from build123d import *

# Parameters (mm, degrees)
BOSS_EXTRUDE1_DEPTH     = 7
CUT_EXTRUDE1_DEPTH      = 3
CUT_EXTRUDE2_DEPTH      = 59.755326779
CUT_EXTRUDE2_DEPTH_BACK = 1
SKETCH5_W               = 5.5
SKETCH5_H               = 5.5
BOSS_EXTRUDE2_DEPTH     = 7
CUT_LOFT3_START         = -28.140767726
CUT_LOFT3_DEPTH         = 25.989204331


# Read off the part's stored shape, not the designer's step: Cut-Loft3
with BuildPart() as part:
    # Sketch1 → Boss-Extrude1 (new body)
    with BuildSketch(Plane(origin=(0, 0, 0), x_dir=(1, 0, 0), z_dir=(0, 1, 0))):
        with BuildLine():
            Line((-56.7108806, 8.042770274), (-56.7108806, 6.805307476))
            Line((-56.7108806, 6.805307476), (51.827852841, 6.805307476))
            Line((51.827852841, 6.805307476), (51.827852841, 8.042770274))
            add(Edge.make_bspline(
                [(51.827852841, 8.042770274), (43.440678216, 9.870534091), (30.144344491, 11.93787877), (11.99631981, 12.860332352), (2.722791962, 12.844934175), (-2.44151388, 12.817702683)],
                knots=[0, 0, 0, 0, 0.47203113, 0.735860593, 1, 1, 1, 1], degree=3))
            add(Edge.make_bspline(
                [(-56.7108806, 8.042770274), (-48.323705975, 9.870534091), (-35.02737225, 11.93787877), (-16.87934757, 12.860332352), (-7.605819721, 12.844934175), (-2.44151388, 12.817702683)],
                knots=[0, 0, 0, 0, 0.47203113, 0.735860593, 1, 1, 1, 1], degree=3))
        make_face()
        with BuildLine():
            Line((51.827852841, 6.805307476), (-56.7108806, 6.805307476))
            Line((-56.7108806, 6.805307476), (-56.7108806, -1.957229726))
            add(Edge.make_bspline(
                [(-56.7108806, -1.957229726), (-48.323705975, -0.129465909), (-35.02737225, 1.93787877), (-16.87934757, 2.860332352), (-7.605819721, 2.844934175), (-2.44151388, 2.817702683)],
                knots=[0, 0, 0, 0, 0.47203113, 0.735860593, 1, 1, 1, 1], degree=3))
            add(Edge.make_bspline(
                [(51.827852841, -1.957229726), (43.440678216, -0.129465909), (30.144344491, 1.93787877), (11.99631981, 2.860332352), (2.722791962, 2.844934175), (-2.44151388, 2.817702683)],
                knots=[0, 0, 0, 0, 0.47203113, 0.735860593, 1, 1, 1, 1], degree=3))
            Line((51.827852841, -1.957229726), (51.827852841, 6.805307476))
        make_face()
        with BuildLine():
            add(Edge.make_bspline(
                [(-56.7108806, -1.957229726), (-48.323705975, -0.129465909), (-35.02737225, 1.93787877), (-16.87934757, 2.860332352), (-7.605819721, 2.844934175), (-2.44151388, 2.817702683)],
                knots=[0, 0, 0, 0, 0.47203113, 0.735860593, 1, 1, 1, 1], degree=3))
            Line((-56.7108806, -1.957229726), (-56.7108806, -3.957229726))
            add(Edge.make_bspline(
                [(-56.7108806, -3.957229726), (-48.323705975, -2.129465909), (-35.02737225, -0.06212123), (-16.87934757, 0.860332352), (-7.605819721, 0.844934175), (-2.44151388, 0.817702683)],
                knots=[0, 0, 0, 0, 0.47203113, 0.735860593, 1, 1, 1, 1], degree=3))
            add(Edge.make_bspline(
                [(51.827852841, -3.957229726), (43.440678216, -2.129465909), (30.144344491, -0.06212123), (11.99631981, 0.860332352), (2.722791962, 0.844934175), (-2.44151388, 0.817702683)],
                knots=[0, 0, 0, 0, 0.47203113, 0.735860593, 1, 1, 1, 1], degree=3))
            Line((51.827852841, -3.957229726), (51.827852841, -1.957229726))
            add(Edge.make_bspline(
                [(51.827852841, -1.957229726), (43.440678216, -0.129465909), (30.144344491, 1.93787877), (11.99631981, 2.860332352), (2.722791962, 2.844934175), (-2.44151388, 2.817702683)],
                knots=[0, 0, 0, 0, 0.47203113, 0.735860593, 1, 1, 1, 1], degree=3))
        make_face()
        with BuildLine():
            Line((-56.7108806, 10.042770274), (-56.7108806, 8.042770274))
            add(Edge.make_bspline(
                [(-56.7108806, 8.042770274), (-48.323705975, 9.870534091), (-35.02737225, 11.93787877), (-16.87934757, 12.860332352), (-7.605819721, 12.844934175), (-2.44151388, 12.817702683)],
                knots=[0, 0, 0, 0, 0.47203113, 0.735860593, 1, 1, 1, 1], degree=3))
            add(Edge.make_bspline(
                [(51.827852841, 8.042770274), (43.440678216, 9.870534091), (30.144344491, 11.93787877), (11.99631981, 12.860332352), (2.722791962, 12.844934175), (-2.44151388, 12.817702683)],
                knots=[0, 0, 0, 0, 0.47203113, 0.735860593, 1, 1, 1, 1], degree=3))
            Line((51.827852841, 8.042770274), (51.827852841, 10.042770274))
            add(Edge.make_bspline(
                [(51.827852841, 10.042770274), (43.440678216, 11.870534091), (30.144344491, 13.93787877), (11.99631981, 14.860332352), (2.722791962, 14.844934175), (-2.44151388, 14.817702683)],
                knots=[0, 0, 0, 0, 0.47203113, 0.735860593, 1, 1, 1, 1], degree=3))
            add(Edge.make_bspline(
                [(-56.7108806, 10.042770274), (-48.323705975, 11.870534091), (-35.02737225, 13.93787877), (-16.87934757, 14.860332352), (-7.605819721, 14.844934175), (-2.44151388, 14.817702683)],
                knots=[0, 0, 0, 0, 0.47203113, 0.735860593, 1, 1, 1, 1], degree=3))
        make_face()
    extrude(amount=BOSS_EXTRUDE1_DEPTH)

    # Sketch3 → Cut-Extrude1 (cut)
    with BuildSketch(Plane(origin=(0, 7, 0), x_dir=(1, 0, 0), z_dir=(0, 1, 0))):
        with BuildLine():
            Line((-54.7108806, 8.868382777), (-54.7108806, -1.931617223))
            add(Edge.make_bspline(
                [(-54.7108806, -1.931617223), (-49.613724747, -0.872437915), (-41.450567172, 0.513475106), (-30.542278229, 1.675797263), (-21.917454503, 2.210860945), (-12.671997291, 2.467388615), (-2.277076443, 2.389216594), (7.816613622, 2.466322462), (17.198414715, 2.202454548), (25.682964859, 1.677700715), (36.725653994, 0.486844708), (44.753602523, -0.877090687), (49.827852841, -1.931574108)],
                knots=[0.018721889, 0.018721889, 0.018721889, 0.018721889, 0.161718627, 0.245988858, 0.319944032, 0.399040882, 0.499999922, 0.605477206, 0.676291886, 0.757771849, 0.838922396, 0.98127786, 0.98127786, 0.98127786, 0.98127786], degree=3))
            Line((49.827852841, -1.931574108), (49.827852841, 8.868425892))
            add(Edge.make_bspline(
                [(-54.7108806, 8.868382777), (-49.613724747, 9.927562085), (-41.450567172, 11.313475106), (-30.542278229, 12.475797263), (-21.917454503, 13.010860945), (-12.671997291, 13.267388615), (-2.277076443, 13.189216594), (7.816613622, 13.266322462), (17.198414715, 13.002454548), (25.682964859, 12.477700715), (36.725653994, 11.286844708), (44.753602523, 9.922909313), (49.827852841, 8.868425892)],
                knots=[0.018721889, 0.018721889, 0.018721889, 0.018721889, 0.161718627, 0.245988858, 0.319944032, 0.399040882, 0.499999922, 0.605477206, 0.676291886, 0.757771849, 0.838922396, 0.98127786, 0.98127786, 0.98127786, 0.98127786], degree=3))
        make_face()
    extrude(amount=-CUT_EXTRUDE1_DEPTH, mode=Mode.SUBTRACT)

    # Sketch5 → Cut-Extrude2 (cut, two sides: drawn at the far end of the back side and taken through both)
    with BuildSketch(Plane(origin=(0, 4, 0), x_dir=(1, 0, 0), z_dir=(0, 1, 0)).offset(-CUT_EXTRUDE2_DEPTH_BACK)):
        with Locations((-49.494843654, 4.328278982)):
            Rectangle(SKETCH5_W, SKETCH5_H)
        with Locations((-39.246490197, 6.065019164)):
            Rectangle(SKETCH5_W, SKETCH5_H)
        with Locations((-28.744225873, 7.063081882)):
            Rectangle(SKETCH5_W, SKETCH5_H)
        with Locations((-18.235416091, 7.740731917)):
            Rectangle(SKETCH5_W, SKETCH5_H)
        with Locations((-7.78097109, 7.938746568)):
            Rectangle(SKETCH5_W, SKETCH5_H)
        with Locations((2.897943331, 7.938746568)):
            Rectangle(SKETCH5_W, SKETCH5_H)
        with Locations((13.352388332, 7.740731917)):
            Rectangle(SKETCH5_W, SKETCH5_H)
        with Locations((23.861198114, 7.063081882)):
            Rectangle(SKETCH5_W, SKETCH5_H)
        with Locations((34.363462438, 6.065019164)):
            Rectangle(SKETCH5_W, SKETCH5_H)
        with Locations((44.611815895, 4.328278982)):
            Rectangle(SKETCH5_W, SKETCH5_H)
    extrude(amount=CUT_EXTRUDE2_DEPTH + CUT_EXTRUDE2_DEPTH_BACK, mode=Mode.SUBTRACT)

    # Sketch6 → Boss-Extrude2 (add)
    with BuildSketch(Plane.XZ):
        Polygon((-56.7108806, -10.042770274), (-56.7108806, -39.797055232), (51.827852841, -39.797055232), (51.827852841, -10.042770274), (-2.44151388, -13.631270719), align=None)
    extrude(amount=-BOSS_EXTRUDE2_DEPTH)

    # Cut-Loft3 outline → Cut-Loft3 (cut)
    with BuildSketch(Plane(origin=(0, 0, 0), x_dir=(1, 0, 0), z_dir=(0, 0.7071067811865518, 0.7071067811865432)).offset(CUT_LOFT3_START)):
        with BuildLine():
            add(Edge.make_bspline(
                [(51.827852841, 12.051058431), (49.604561047, 12.393258463), (45.142487075, 13.027898019), (38.409103261, 13.825796232), (31.641249387, 14.461164843), (24.84585392, 14.933029584), (18.032893375, 15.237107028), (11.210055122, 15.405236678), (4.384500343, 15.443691251), (-2.441535298, 15.418403963), (-9.267454577, 15.445172671), (-16.093054432, 15.404982103), (-22.915912391, 15.237149433), (-29.728909591, 14.933046954), (-36.524242812, 14.461126298), (-43.292105117, 13.825843609), (-50.025574302, 13.027890419), (-54.487633846, 12.393258899), (-56.7108806, 12.051058431)],
                knots=[0.621766015, 0.621766015, 0.621766015, 0.621766015, 0.645405639, 0.669045263, 0.692684887, 0.716324512, 0.739964136, 0.76360376, 0.787243384, 0.810883008, 0.834522632, 0.858162256, 0.88180188, 0.905441504, 0.929081128, 0.952720752, 0.976360376, 1, 1, 1, 1], degree=3))
            Line((51.827852841, 12.051058431), (51.827852841, 35))
            Line((51.827852841, 35), (-56.7108806, 35))
            Line((-56.7108806, 35), (-56.7108806, 12.051058431))
        make_face()
    extrude(amount=CUT_LOFT3_DEPTH, mode=Mode.SUBTRACT)


solid = part.part
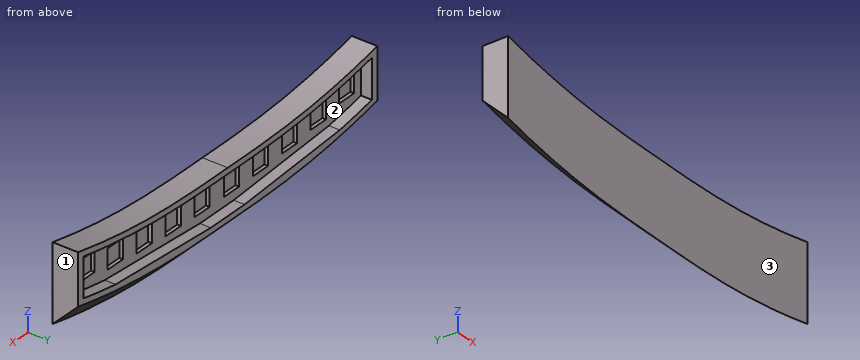
For this review, take the finished solid that the model builds, in its own axes (mm). Face numbers are marked on the shaded views. Coordinates: 2 decimals unless noted, no trailing zeros. Return JSON: item names as keys, results as strings.
1. For pin 1 Ø4 at (x, z) = (-23, -8.5) entering from +Y; pin 2 Ø0.5 at (x, y) = (12, 3.5) entering from -Z; pin 3 Ø1.6 at (x, z) = (-48, -3.5) entering from +Y, all flat-tipped, find the tip position at first contact; note any pin that passes through.
Answer block:
{"pin 1": "y = 4", "pin 2": "z = -18.49", "pin 3": "y = 3"}
2. For line 1 (X direction, y = 5, z = -4); line 2 (Y direction, x = -50.5, z = 0); line 3 (Y direction, x = 46, z = -2), list the stretches that pass through material, from the lowest coordinate up. Write a range as from..to.
Answer block:
{"line 1": "-56.71..-54.71, 49.83..51.83", "line 2": "0..4", "line 3": "0..3"}
3. The part is to be moulded in two halves that separate along X. For the marked faces 1, 2 and 3, say which applies: +X half, -X half, draft (parallel to the pull), parting line (faces both ways), or undercut.
Answer block:
{"face 1": "+X half", "face 2": "undercut", "face 3": "draft"}
